from build123d import *

# Parameters (mm, degrees)
SKETCH1_R                = 7.051488697
BOSS_EXTRUDE1_DEPTH      = 3
SKETCH2_R                = 7.051488697
BOSS_EXTRUDE2_DEPTH      = 4
SKETCH3_R                = 3.75
CUT_EXTRUDE1_DEPTH       = 93.010868923
CUT_EXTRUDE2_START       = -3
CUT_EXTRUDE2_DEPTH       = 1.5
SKETCH5_W                = 67.326740962
SKETCH5_H                = 77.001413362
CUT_EXTRUDE4_DEPTH       = 6
BOSS_EXTRUDE3_DEPTH      = 10
BOSS_EXTRUDE3_DEPTH_BACK = 1
SKETCH6_W                = 13
SKETCH6_H                = 26.261119779
CUT_EXTRUDE5_DEPTH       = 89.770385235


with BuildPart() as part:
    # Sketch1 → Boss-Extrude1 (new body)
    with BuildSketch(Plane(origin=(0, 0, 0), x_dir=(1, 0, 0), z_dir=(0, 1, 0))):
        with BuildLine():
            Line((6.693069307, -1.487522855), (6.693069307, -51.567458957))
            ThreePointArc((6.693069307, -51.567458957), (22.956358252, -46.658392769), (36.769552622, -36.769552622))
            ThreePointArc((36.769552622, -36.769552622), (43.25852742, -28.856538348), (48.072152744, -19.825945893))
            Line((48.072152744, -19.825945893), (60.09019093, -24.782432367))
            ThreePointArc((60.09019093, -24.782432367), (54.073159275, -36.070672935), (45.961940777, -45.961940777))
            ThreePointArc((45.961940777, -45.961940777), (26.581470301, -59.316316783), (3.715889133, -64.893698985))
            ThreePointArc((3.715889133, -64.893698985), (0.18200985, -64.999745172), (-3.352407903, -64.913491365))
            ThreePointArc((-3.352407903, -64.913491365), (-7.908445684, -59.104066137), (-5.814964059, -52.024218933))
            Line((-5.814964059, -52.024218933), (-5.814964059, -3.088434015))
            Line((-5.814964059, -3.088434015), (-5.814964059, 3.911565985))
            Line((-5.814964059, 3.911565985), (-5.814964059, 6.911565985))
            Line((-5.814964059, 6.911565985), (6.693069307, 6.911565985))
            Line((6.693069307, 6.911565985), (6.693069307, 3.911565985))
            Line((6.693069307, 3.911565985), (6.693069307, -1.487522855))
        make_face()
        with Locations(Location((0, -57.593120372, 0), (0, 0, 270))):
            Circle(SKETCH1_R, mode=Mode.SUBTRACT)
    extrude(amount=BOSS_EXTRUDE1_DEPTH)

    # Sketch2 → Boss-Extrude2 (add)
    with BuildSketch(Plane(origin=(0, 3, 0), x_dir=(1, 0, 0), z_dir=(0, 1, 0))):
        with BuildLine():
            Line((-5.814964059, -47.160734717), (6.693069307, -47.160734717))
            Line((6.693069307, -47.160734717), (6.693069307, -51.567458957))
            ThreePointArc((6.693069307, -51.567458957), (31.649459702, -41.259080219), (48.072152744, -19.825945893))
            ThreePointArc((48.072152744, -19.825945893), (51.008587231, -10.105643407), (52, 0))
            Line((52, 0), (65, 0))
            ThreePointArc((65, 0), (63.760734039, -12.632054258), (60.09019093, -24.782432367))
            ThreePointArc((60.09019093, -24.782432367), (34.747942094, -54.932508774), (-3.352407903, -64.913491365))
            ThreePointArc((-3.352407903, -64.913491365), (-7.908445684, -59.104066137), (-5.814964059, -52.024218933))
            Line((-5.814964059, -52.024218933), (-5.814964059, -47.160734717))
        make_face()
        with Locations(Location((0, -57.593120372, 0), (0, 0, 270))):
            Circle(SKETCH2_R, mode=Mode.SUBTRACT)
    extrude(amount=BOSS_EXTRUDE2_DEPTH)

    # Sketch3 → Cut-Extrude1 (cut, through all)
    with BuildSketch(Plane(origin=(0, 3, 0), x_dir=(1, 0, 0), z_dir=(0, 1, 0))):
        with Locations(Location((0, 0, 0), (0, 0, 270))):
            Circle(SKETCH3_R)
    extrude(amount=-CUT_EXTRUDE1_DEPTH, mode=Mode.SUBTRACT)

    # Sketch4 → Cut-Extrude2 (cut)
    with BuildSketch(Plane.XZ.offset(CUT_EXTRUDE2_START)):
        with BuildLine():
            Line((3.75, 0), (1.65, 14))
            ThreePointArc((1.65, 14), (-0.35, 16), (-2.35, 14))
            Line((-2.35, 14), (-3.75, 0))
            ThreePointArc((-3.75, 0), (0, -3.75), (3.75, 0))
        make_face()
    extrude(amount=CUT_EXTRUDE2_DEPTH, mode=Mode.SUBTRACT)

    # Sketch5 → Cut-Extrude4 (cut)
    with BuildSketch(Plane.XZ):
        with Locations((42.047234811, 32.501031374)):
            Rectangle(SKETCH5_W, SKETCH5_H)
    extrude(amount=-CUT_EXTRUDE4_DEPTH, mode=Mode.SUBTRACT)

    # Sketch6 → Boss-Extrude3 (add, two sides: drawn at the far end of the back side and taken through both)
    with BuildSketch(Plane.XZ.offset(-6).offset(-BOSS_EXTRUDE3_DEPTH_BACK)):
        with Locations((58.5, -13.13055989)):
            Rectangle(SKETCH6_W, SKETCH6_H)
    extrude(amount=BOSS_EXTRUDE3_DEPTH + BOSS_EXTRUDE3_DEPTH_BACK)

    # Sketch7 → Cut-Extrude5 (cut, through all)
    with BuildSketch(Plane.ZY.offset(-52)):
        Polygon((0, 7), (-26.261119779, 1.5), (-26.261119779, 7), align=None)
        Polygon((-26.261119779, 0.5), (0, 6), (0, -4), (-26.261119779, -4), align=None)
    extrude(amount=-CUT_EXTRUDE5_DEPTH, mode=Mode.SUBTRACT)


solid = part.part
Source: CAD feature listing. Evaluate the final solid. Frame: model axes, mm. A direction names the side the tool comes from. Coordinates: 2 decimals unless noted, no trailing zeros. Write each loop counter-clockwise with the first axis right and the second up, starting at its lowest first coordinate (ties: lowest second). Pieces come first, ordered by that corner, then holes. Notation, with made-up numbers: M 23.5,82.5 L 57.5,82.5 A19 cw 57.5,95.5 Z; hole C 76.5,54 d5. An arc over 180 degrees is marked long. Use a Markdown table: item, result.
1) Section C-C, the plane x = 0. Output: boundary loops of the cut face in (y, z), then the cut area to 3 significant figures.
Conclusion:
| item | result |
|---|---|
| outline | M 0,-6.91 L 3,-6.91 L 3,-3.75 L 0,-3.75 Z; M 0,3.75 L 1.5,3.75 L 1.5,15.97 L 3,15.97 L 3,47.16 L 7,47.16 L 7,50.54 L 0,50.54 Z; M 0,64.64 L 7,64.64 L 7,65 L 0,65 Z |
| area | 148 mm^2 |
2) Section A-A, the plane y = 4. Output: boundary loops of the cut face in (x, z).
Conclusion:
| item | result |
|---|---|
| outline | M -5.81,47.16 L 6.69,47.16 L 6.69,51.57 A52 cw 8.38,51.32 L 8.38,64.46 A65 ccw -3.35,64.91 A8.05 ccw -5.81,52.02 Z; M 52,-14.32 L 65,-14.32 L 65,-9.55 L 52,-9.55 Z; hole C 0,57.59 d14.1 |
3) Reachability of faces 4 (the flat face through (0, 5, 47.161)), 5 (the flat face through (41, 6, 37)), 6 (the flat face through (8.384, 3, 58)), 7 (the flat face through (1, 3, 20)) from +Z, -Z, +X, -X, +Y, -Y: full face, straight path, thin tool, end or side. Return the list, or none.
Conclusion:
| item | result |
|---|---|
| face 4 | -Z, -X, +Y |
| face 5 | +Z, +X, -Y |
| face 6 | +Z, -Z, +X, -Y |
| face 7 | -Z, +X, -X, +Y |
4) Section D-D, the plane x = 21.5. Output: boundary loops of the cut face in (y, z), then the cut area to 3 significant figures.
Conclusion:
| item | result |
|---|---|
| outline | M 6,47.35 L 7,47.35 L 7,61.34 L 6,61.34 Z |
| area | 14.0 mm^2 |
5) Mould query, pull axis X, two halves, no side actions, for faces 1 (the cylindrical face through (-7.888, 3.451, 59.209)), 2 (the flat face through (58.409, 3.212, -13.314)), 3 (the cylindrical face through (0.31, 3.45, 50.55)). Classes: pulls with the +X half, pulls with the -X half, needs draft (parallel to the pull), parting line crosses it, or undercut.
Conclusion:
| item | result |
|---|---|
| face 1 | pulls with the -X half |
| face 2 | needs draft |
| face 3 | undercut |
6) Section B-B, the plane z = 15. Output: boundary loops of the cut face in (x, y).
Conclusion:
| item | result |
|---|---|
| outline | M -5.81,0 L 6.69,0 L 6.69,3 L 1.38,3 L 1.38,1.5 L -2.08,1.5 L -2.08,3 L -5.81,3 Z; M 49.79,6 L 63.25,6 L 63.25,7 L 49.79,7 Z |
7) First-contact query: pin 1 Ø8 at (x, z) = (-1, 11) entering from +Y; pin 2 Ø17 at (x, z) = (27.5, 39) entering from -Y; pin 3 Ø3.5 at (y, z) = (2, 26) entering from +X. Flat tips, straight axial feed; report the tip coordinate or a pass-through.
Conclusion:
| item | result |
|---|---|
| pin 1 | stops at y = 3 |
| pin 2 | stops at y = 6 |
| pin 3 | stops at x = 6.69 |
8) Ray query, L1, parallel to X at y = 1.6, z = 0; L2, parallel to X at y = 5.25, z = 57; L3, parallel to X at y = 2, z = 23. Return the intervals inside material, ascending.
Conclusion:
| item | result |
|---|---|
| L1 | x = -5.81 to -3.75, 3.75 to 6.69 |
| L2 | x = -8.03 to -7.03, 7.03 to 8.38 |
| L3 | x = -5.81 to 6.69 |
